The figure shows three views and two pictorial views of one solid part (mm, origin at its lowest corner). Answer the questions. Give positions to 0.01 mm unless a question says otherwise; leave off trailing zeros. Order: outer loops, then holes, each group sorted by start corner. A loop starts at its lowest first (then second) coordinate and runs counter-clockwise, first axis right, second up. Notation, with made-up numbers: M 59.5,86 L 85.5,86 A11 cw 85.5,99 Z; hole C 73,81.5 d4. An arc over 180 degrees is marked long. One line per item, written item: value. Start each with the question number.
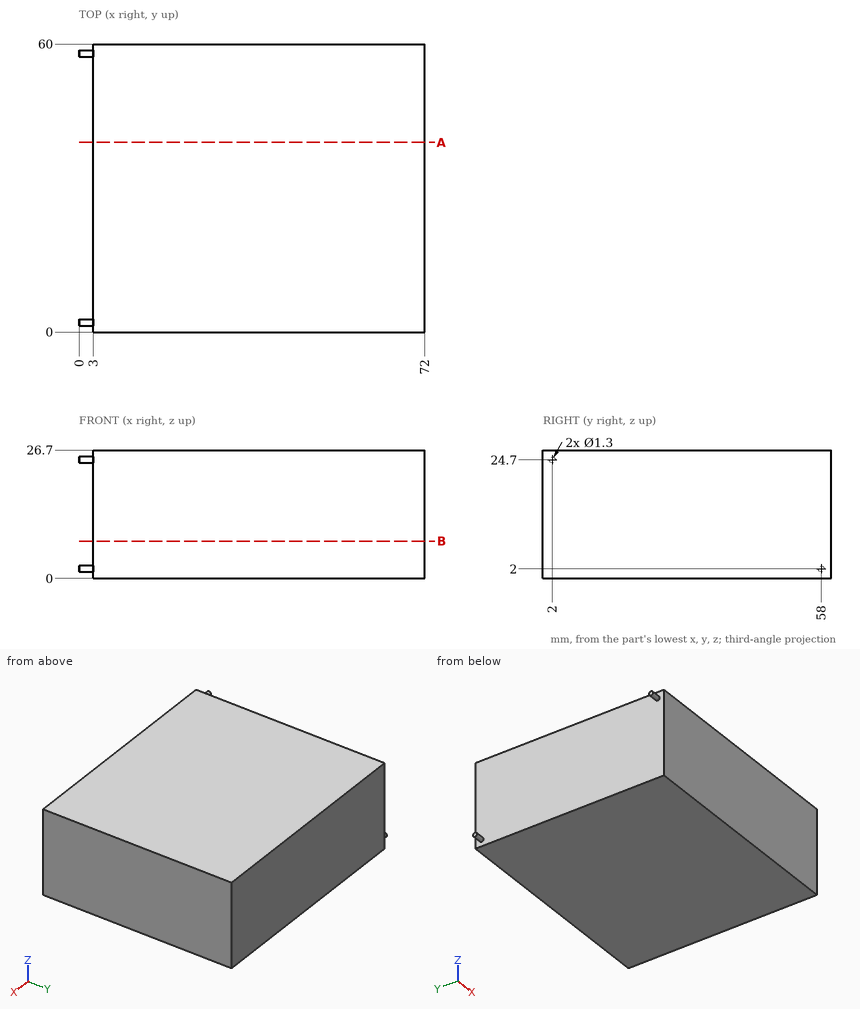
Q1. Find section A-A, the plane y = 39.5. Give the vertices of the cut face in (x, z), then the cut area to 3 significant figures.
Q2. Consider probe 1 along X at (y, z) = (42.5, 16.5). Determine where the line is inside the solid, lowest interval first.
Q3. Find section B-B, the plane z = 7.75. Give the vertices of the cut face in (x, y), then the cut area to 3 significant figures.
Evaluation:
1. outline: M 3,0 L 72,0 L 72,26.7 L 3,26.7 Z
1. area: 1,840 mm2
2. probe 1: 3 to 72
3. outline: M 3,0 L 72,0 L 72,60 L 3,60 Z
3. area: 4,140 mm2
